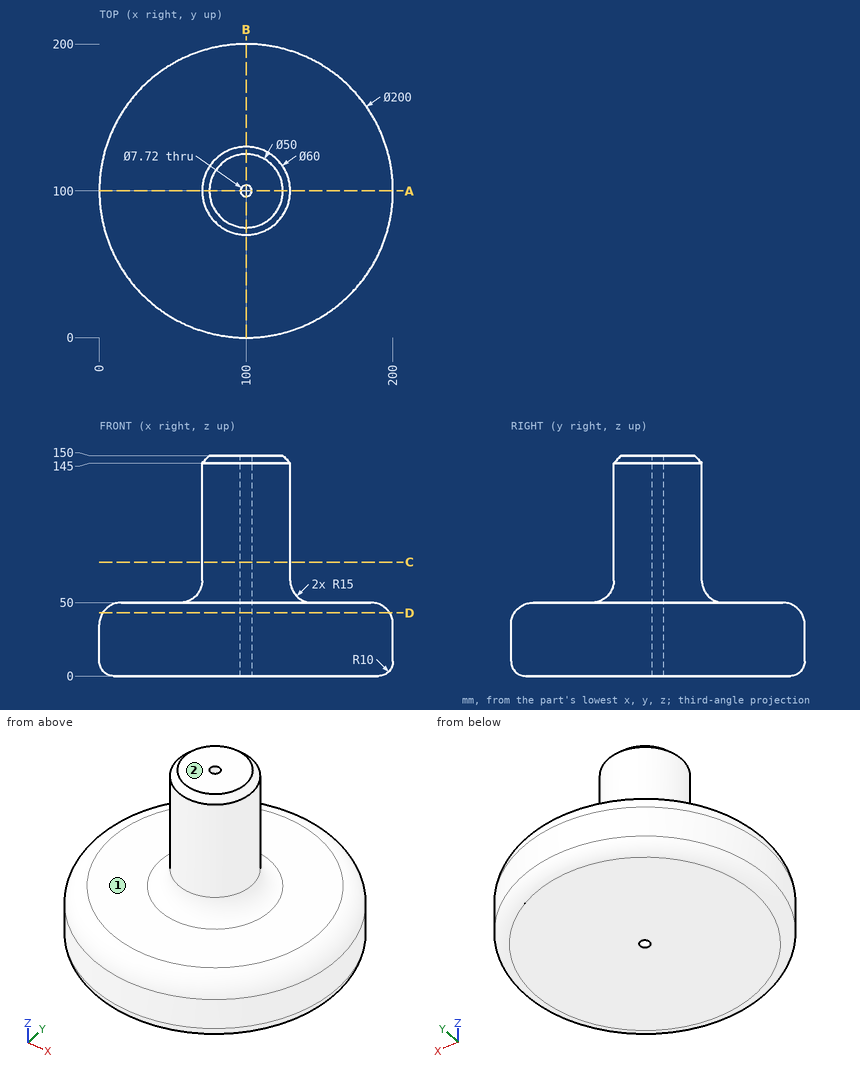
The drawing under review shows one solid part. Ordinate dimensions are in mm from its lowest x, y, z. A direction names the side the tool comes from. Coordinates: 2 decimals unless noted, no trailing zeros. Write each loop counter-clockwise with the first axis right and the second up, starting at its lowest first coordinate (ties: lowest second). Pieces come first, ordered by that corner, then holes. Notation, with made-up numbers: (18, -28.5) - (74, -28.5) arc R11 ccw to (74, -15.5) - close; hole circle Ø7 at (73.5, -3). An arc over 180 degrees is marked (long way). Put each result on its own line as item: value.
1. Wall thickness on probe 1 along Y at (x, z) = (100, 111); probe 2 along Y at (x, z) = (100, 31.5); probe 3 along Z at (x, y) = (50.5, 141.5): over which ranges is each line inside the solid? List them lowest first.
Values found:
probe 1: 70 to 96.14, 103.86 to 130
probe 2: 0 to 96.14, 103.86 to 200
probe 3: 0 to 50
2. Add section A-A, the plane y = 100. Give the boundary of the cut face in (x, z), then the cut area to 3 significant figures.
Values found:
outline: (0, 10) arc R10 ccw to (10, 0) - (96.14, 0) - (96.14, 150) - (75, 150) - (70, 145) - (70, 65) arc R15 cw to (55, 50) - (15, 50) arc R15 ccw to (0, 35) - close; (103.86, 0) - (190, 0) arc R10 ccw to (200, 10) - (200, 35) arc R15 ccw to (185, 50) - (145, 50) arc R15 cw to (130, 65) - (130, 145) - (125, 150) - (103.86, 150) - close
area: 14,800 mm²
3. For pin 1 (1 mm diameter, centred on x = 102.5, z = 80.5, fed in from -Y); pin 2 (1 mm diameter, centred on x = 26.5, y = 111.5, fed in from -Z); pin 3 (12 mm diameter, centred on x = 83.5, z = 84, fed in from -Y); pin 4 (2 mm diameter, centred on x = 52, z = 27.5, fed in from -Y), all flat-tipped, find the tip position at first contact; note any pin that passes through.
Values found:
pin 1: y = 70.07
pin 2: z = 0
pin 3: y = 71.9
pin 4: y = 11.73
4. Machinability: for the marked faces 1 and 2, which of the approach directions +Z, -Z, +X, -X, +Y, -Y give a long, thin tool a straight path to every point of the face, cutting with its end or side? Answer none if there is none.
Values found:
face 1: +Z
face 2: +Z, +X, -X, +Y, -Y
5. Add section D-D, the plane z = 43. Give the boundary of the cut face in (x, y), then the cut area to 3 significant figures.
Values found:
outline: circle Ø195.38 at (100, 100); hole circle Ø7.72 at (100, 100)
area: 29,900 mm²
6. Add section C-C, the plane z = 77.5. Give the boundary of the cut face in (x, y), then the cut area to 3 significant figures.
Values found:
outline: circle Ø60 at (100, 100); hole circle Ø7.72 at (100, 100)
area: 2,780 mm²
